Can you work these out from the model? Positions are in its coordinate system, mm. A direction names the side the tool comes from. Give positions to 0.01 mm unless a question says otherwise; leave off trailing zeros. Loops run counter-clockwise (first coordinate to the right, second up) from the corner with the lowest first, then second, coordinate; pieces in that order, holes last. Notation, with made-up numbers: M 71,87.25 L 101,87.25 A26 ccw 101,124.25 Z; hole C -14.75,8.25 d8. An arc over 180 degrees is marked long. Answer as a JSON object with one key per item and string values.
```python
from build123d import *

# Parameters (mm, degrees)
F0_W     = 254
F0_H     = 254
F6_DEPTH = 127
F7_W     = 50.8
F7_H     = 50.8
F1_DEPTH = 254.001
F2_W     = 50.8
F2_H     = 50.8
F3_DEPTH = 254.001
F4_W     = 50.8
F4_H     = 50.8
F8_DEPTH = 254.001
F9_R     = 12.7


with BuildPart() as f6:
    # F0 (on Front) → F6 (new body, symmetric)
    with BuildSketch(Plane.XZ):
        Rectangle(F0_W, F0_H)
    extrude(amount=F6_DEPTH, both=True)

    # F7 (on face) → F1 (cut, through all)
    with BuildSketch(Plane(origin=(0, 0, -127), x_dir=(1, 0, 0), z_dir=(0, 0, -1))):
        Rectangle(F7_W, F7_H)
    extrude(amount=-F1_DEPTH, mode=Mode.SUBTRACT)

    # F2 (on face) → F3 (cut, through all)
    with BuildSketch(Plane.YZ.offset(127)):
        Rectangle(F2_W, F2_H)
    extrude(amount=-F3_DEPTH, mode=Mode.SUBTRACT)

    # F4 (on face) → F8 (cut, through all)
    with BuildSketch(Plane(origin=(0, 127, 0), x_dir=(-1, 0, 0), z_dir=(0, 1, 0))):
        Rectangle(F4_W, F4_H)
    extrude(amount=-F8_DEPTH, mode=Mode.SUBTRACT)

    # F9
    f9_edges = [f6.edges().sort_by_distance(p)[0] for p in [
        (127, 127, 0),
        (127, 0, -127),
        (127, 0, 127),
        (127, -127, 0),
        (127, 25.4, 0),
        (127, 0, 25.4),
        (127, -25.4, 0),
        (127, 0, -25.4),
        (0, -127, -127),
        (0, -127, 127),
        (-127, -127, 0),
        (-25.4, -127, 0),
        (0, -127, -25.4),
        (25.4, -127, 0),
        (0, -127, 25.4),
        (-127, 0, 127),
        (-127, 127, 0),
        (-127, 0, -127),
        (-127, 25.4, 0),
        (-127, 0, -25.4),
        (-127, -25.4, 0),
        (-127, 0, 25.4),
        (0, 127, -127),
        (0, 127, 127),
        (0, 127, -25.4),
        (25.4, 127, 0),
        (0, 127, 25.4),
        (-25.4, 127, 0),
        (25.4, 0, 127),
        (0, 25.4, 127),
        (-25.4, 0, 127),
        (0, -25.4, 127),
        (25.4, 0, -127),
        (0, -25.4, -127),
        (-25.4, 0, -127),
        (0, 25.4, -127),
    ]]
    fillet(f9_edges, radius=F9_R)


solid = f6.part
```
1) For faces 1 (the flat face through (-69, 0, -25.4)), 2 (the cylindrical face through (-0.53, 123.38, -29.22)), 3 (the flat face through (-25.4, 70, 0)), which set-ups out of +Z, -Z, +X, -X, +Y, -Y let a thin tool reach every point of the face, with its end or its side?
Answer list:
{"face 1": "+X, -X", "face 2": "+Y", "face 3": "+Y, -Y"}
2) Suppose I cut it at B-B, the plane y = 54. Write out the boundary of the cut face in (x, z), and give its area (3 significant figures).
Answer list:
{"outline": "M -127,-114.3 A12.7 ccw -114.3,-127 L 114.3,-127 A12.7 ccw 127,-114.3 L 127,114.3 A12.7 ccw 114.3,127 L -114.3,127 A12.7 ccw -127,114.3 Z; hole M -25.4,-25.4 L 25.4,-25.4 L 25.4,25.4 L -25.4,25.4 Z", "area": "61,800 mm^2"}
3) Suppose I cut it at A-A, the plane x = -4. Write out the boundary of the cut face in (y, z), and give its area (3 significant figures).
Answer list:
{"outline": "M -127,-114.3 A12.7 ccw -114.3,-127 L -38.1,-127 A12.7 ccw -25.4,-114.3 L -25.4,-25.4 L -114.3,-25.4 A12.7 ccw -127,-38.1 Z; M -127,38.1 A12.7 ccw -114.3,25.4 L -25.4,25.4 L -25.4,114.3 A12.7 ccw -38.1,127 L -114.3,127 A12.7 ccw -127,114.3 Z; M 25.4,-114.3 A12.7 ccw 38.1,-127 L 114.3,-127 A12.7 ccw 127,-114.3 L 127,-38.1 A12.7 ccw 114.3,-25.4 L 25.4,-25.4 Z; M 25.4,25.4 L 114.3,25.4 A12.7 ccw 127,38.1 L 127,114.3 A12.7 ccw 114.3,127 L 38.1,127 A12.7 ccw 25.4,114.3 Z", "area": "40,900 mm^2"}
4) If we mould it in two halves opening along Y, with no side actions, what happens to faces 4 (the flat face through (25.4, 70, 0)), 5 (the cylindrical face through (29.22, -0.53, 123.38)), 6 (the cylindrical face through (1.6, 123.18, -123.38))? For each: +Y half, -Y half, draft (parallel to the pull), parting line (faces both ways), or undercut.
Answer list:
{"face 4": "draft", "face 5": "undercut", "face 6": "+Y half"}
5) Please list where this line runs through material, in increasing order: line 1 along X through (y, z) = (0, 75.5). Write a range as from..to.
Answer list:
{"line 1": "-127..-25.4, 25.4..127"}
6) Suppose I cut it at D-D, the plane x = -31. Write out the boundary of the cut face in (y, z), and give its area (3 significant figures).
Answer list:
{"outline": "M -127,-114.3 A12.7 ccw -114.3,-127 L -38.1,-127 A12.7 ccw -31,-124.83 L 31,-124.83 A12.7 ccw 38.1,-127 L 114.3,-127 A12.7 ccw 127,-114.3 L 127,-38.1 A12.7 ccw 124.83,-31 L 124.83,31 A12.7 ccw 127,38.1 L 127,114.3 A12.7 ccw 114.3,127 L 38.1,127 A12.7 ccw 31,124.83 L -31,124.83 A12.7 ccw -38.1,127 L -114.3,127 A12.7 ccw -127,114.3 L -127,38.1 A12.7 ccw -124.83,31 L -124.83,-31 A12.7 ccw -127,-38.1 Z; hole M -25.4,-25.4 L 25.4,-25.4 L 25.4,25.4 L -25.4,25.4 Z", "area": "61,200 mm^2"}
7) Will this pin go through, and if not, where does the flat tip stop? pin 1 Ø2 at (y, z) = (28, 2) entering from +X.
Answer list:
{"pin 1": "x = 123.16"}
